from build123d import *

# Parameters (mm, degrees)
F0_W     = 24.5
F0_H     = 10
F0_R     = 1.5
F0_W_2   = 8.5
F1_DEPTH = 1
F2_W     = 6.5
F2_H     = 6.4
F2_R     = 1.5
F2_W_2   = 3
F3_DEPTH = 3
F2_W_3   = 4.25
F4_DEPTH = 11
F5_W     = 5.7
F5_H     = 10
F6_DEPTH = 7


with BuildPart() as f1:
    # F0 (on Top) → F1 (new body)
    with BuildSketch(Plane.XY):
        Rectangle(F0_W, F0_H)
        with Locations((-9.5, 0)):
            Circle(F0_R, mode=Mode.SUBTRACT)
        with Locations((9.5, 0)):
            Circle(F0_R, mode=Mode.SUBTRACT)
        with Locations((16.5, 0)):
            Rectangle(F0_W_2, F0_H)
    extrude(amount=F1_DEPTH)

    # F2 (on face) → F3 (join)
    with BuildSketch(Plane.XY.offset(1)):
        with Locations((-9, 0)):
            Rectangle(F2_W, F2_H)
        with Locations((-9.5, 0)):
            Circle(F2_R, mode=Mode.SUBTRACT)
        Rectangle(F2_W_2, F2_H)
        with Locations((9, 0)):
            Rectangle(F2_W, F2_H)
        with Locations((9.5, 0)):
            Circle(F2_R, mode=Mode.SUBTRACT)
    extrude(amount=F3_DEPTH)

    # F2 (on face) → F4 (join)
    with BuildSketch(Plane.XY.offset(1)):
        with Locations((-3.625, 0)):
            Rectangle(F2_W_3, F2_H)
        with Locations((3.625, 0)):
            Rectangle(F2_W_3, F2_H)
    extrude(amount=F4_DEPTH)

    # F5 (on face) → F6 (join)
    with BuildSketch(Plane(origin=(0, 0, 0), x_dir=(1, 0, 0), z_dir=(0, 0, -1))):
        with Locations((17.9, 0)):
            Rectangle(F5_W, F5_H)
    extrude(amount=F6_DEPTH)


solid = f1.part
The listing builds one solid part. Answer for the finished solid, in the listing's coordinates (mm). A direction names the side the tool comes from. Coordinates: 2 decimals unless noted, no trailing zeros. Loops run counter-clockwise (first coordinate to the right, second up) from the corner with the lowest first, then second, coordinate; pieces in that order, holes last.
1) Find section D-D on y = -2. Write down the section's boundary in (x, z), then the cut area to 3 significant figures.
2) Find section B-B on x = -9.5. Write down the section's boundary in (y, z), then the cut area to 3 significant figures.
3) Find section C-C on z = 2.25. Write down the section's boundary in (x, y), then the cut area to 3 significant figures.
4) A tool of negligible diameter and unlimited length cuts with its end or side. For faces 1 (the face through (-1.5, 0, 8)), 2 (the face through (-5.75, 0, 8)), 3 (the face through (1, 0, 0)), 4 (the face through (7.5, 0, 4)), from which of +Z, -Z, +X, -X, +Y, -Y can it reach the whole face along a straight path? Write none if from no direction.
5) Find section A-A on y = 0. Write down the section's boundary in (x, z).
6) Flat-ended cylindrical pins translate along their axes: pin 1 Ø0.9 at (y, z) = (0, 3) entering from +X; pin 2 Ø2.5 at (x, y) = (0.5, 0) entering from +Z; pin 3 Ø3.5 at (x, z) = (-2.5, 7.5) entering from -Y; pin 4 Ø3 at (y, z) = (0.5, 6.5) entering from +X. Find the tip coordinate at first contact, or state that the pin passes through.
7) Find the intervals of material crossed by L1, parallel to X at y = 3, z = 7.75; L2, parallel to Y at x = 9.5, z = 1.65; L3, parallel to X at y = -4.5, z = -4, in increasing order.
8) Determine the mould class of faces 5 (the face through (0, -3.2, 3)), 6 (the face through (-11, 0, 2)), 7 (the face through (5.75, 0, 8)) for opening direction Y: pulls with the +Y half, pulls with the -Y half, needs draft (parallel to the pull), parting line crosses it, or undercut.
Values:
1. outline: (-12.25, 0) - (15.05, 0) - (15.05, -7) - (20.75, -7) - (20.75, 1) - (12.25, 1) - (12.25, 4) - (5.75, 4) - (5.75, 12) - (1.5, 12) - (1.5, 4) - (-1.5, 4) - (-1.5, 12) - (-5.75, 12) - (-5.75, 4) - (-12.25, 4) - close
1. area: 214 mm2
2. outline: (-5, 0) - (-1.5, 0) - (-1.5, 4) - (-3.2, 4) - (-3.2, 1) - (-5, 1) - close; (1.5, 0) - (5, 0) - (5, 1) - (3.2, 1) - (3.2, 4) - (1.5, 4) - close
2. area: 17.2 mm2
3. outline: (-12.25, -3.2) - (12.25, -3.2) - (12.25, 3.2) - (-12.25, 3.2) - close; hole circle Ø3 at (-9.5, 0); hole circle Ø3 at (9.5, 0)
3. area: 143 mm2
4. face 1: +Z, +Y, -Y
4. face 2: +Z, -X, +Y, -Y
4. face 3: -Z, -X, +Y, -Y
4. face 4: +Z, +X, +Y, -Y
5. outline: (-12.25, 0) - (-11, 0) - (-11, 4) - (-12.25, 4) - close; (-8, 0) - (8, 0) - (8, 4) - (5.75, 4) - (5.75, 12) - (1.5, 12) - (1.5, 4) - (-1.5, 4) - (-1.5, 12) - (-5.75, 12) - (-5.75, 4) - (-8, 4) - close; (11, 0) - (15.05, 0) - (15.05, -7) - (20.75, -7) - (20.75, 1) - (12.25, 1) - (12.25, 4) - (11, 4) - close
6. pin 1: stops at x = 12.25
6. pin 2: stops at z = 12
6. pin 3: stops at y = -3.2
6. pin 4: stops at x = 5.75
7. L1: x = -5.75 to -1.5, 1.5 to 5.75
7. L2: y = -3.2 to -1.5, 1.5 to 3.2
7. L3: x = 15.05 to 20.75
8. face 5: pulls with the -Y half
8. face 6: undercut
8. face 7: needs draft
